Could you check a few things on this model? Use its own coordinates, in mm. A direction names the side the tool comes from. Coordinates: 2 decimals unless noted, no trailing zeros. Write each loop counter-clockwise with the first axis right and the second up, starting at its lowest first coordinate (ties: lowest second). Pieces come first, ordered by that corner, then holes.
Item 1: I want a section at A-A on z = -119. Please give me the cut outline in (x, y).
Item 2: If I drill on probe 1 along Z at (x, y) = (85.5, 527); probe 2 along Y at (x, z) = (212.5, -297.5), over which ranges is the centre line in solid material (lowest first)?
Item 3: I want a section at D-D on x = -209. Please give me the cut outline in (y, z), then the cut area to 3 significant figures.
Item 4: I want a section at C-C on x = 107. Please give me the cut outline in (y, z), then the cut area to 3 significant figures.
Item 5: I want a section at B-B on y = 388. Please give me the cut outline in (x, z).
Item 6: Thinking about a two-plate mould opening in Y: for faces 5 (the flat face through (190.5, 27, -150)), 6 (the flat face through (3, 313, 330.2)), 7 (the flat face through (3, 313, -330.2)), 8 (the flat face through (-218, 0, 5)), which applies, +Y half, -Y half, draft (parallel to the pull), parting line (faces both ways), or undercut?
Item 7: Which directions (+Z, -Z, +X, -X, +Y, -Y) give clear straight access to the entire face, cutting with the end or side of a thin tool? Please do faces 1 (the flat face through (-190.5, 611, 201)), 2 (the flat face through (216, 588.496, -155)), 3 (the flat face through (3, 313, 25.4)), 4 (the flat face through (3, 313, 381)).
from build123d import *

# Parameters (mm, degrees)
F0_W     = 381
F0_H     = 50.8
F0_W_2   = 50.8
F1_DEPTH = 635
F2_W     = 533.4
F2_H     = 254
F2_H_2   = 355.6
F3_DEPTH = 482.601


with BuildPart() as f1:
    # F0 (on Front) → F1 (new body)
    with BuildSketch(Plane.XZ):
        with Locations((0, 355.6)):
            Rectangle(F0_W, F0_H)
        Polygon((241.3, 381), (190.5, 381), (190.5, 330.2), (190.5, 76.2), (241.3, 76.2), align=None)
        Polygon((241.3, 25.4), (190.5, 25.4), (190.5, -330.2), (190.5, -381), (241.3, -381), align=None)
        with Locations((0, -355.6)):
            Rectangle(F0_W, F0_H)
        Polygon((-190.5, 381), (-241.3, 381), (-241.3, 76.2), (-190.5, 76.2), (-190.5, 330.2), align=None)
        Polygon((-190.5, 25.4), (-241.3, 25.4), (-241.3, -381), (-190.5, -381), (-190.5, -330.2), align=None)
        with Locations((0, 50.8)):
            Rectangle(F0_W, F0_H)
        with Locations((-215.9, 50.8)):
            Rectangle(F0_W_2, F0_H)
        with Locations((215.9, 50.8)):
            Rectangle(F0_W_2, F0_H)
    extrude(amount=-F1_DEPTH)

    # F2 (on face) → F3 (cut, through all)
    with BuildSketch(Plane.YZ.offset(241.3)):
        with Locations((321.7956796288, 203.2)):
            Rectangle(F2_W, F2_H)
        with Locations((321.7956796288, -152.4)):
            Rectangle(F2_W, F2_H_2)
    extrude(amount=-F3_DEPTH, mode=Mode.SUBTRACT)


solid = f1.part
Response values:
1. outline: (-241.3, 0) - (-190.5, 0) - (-190.5, 55.1) - (-241.3, 55.1) - close; (-241.3, 588.5) - (-190.5, 588.5) - (-190.5, 635) - (-241.3, 635) - close; (190.5, 0) - (241.3, 0) - (241.3, 55.1) - (190.5, 55.1) - close; (190.5, 588.5) - (241.3, 588.5) - (241.3, 635) - (190.5, 635) - close
2. probe 1: z = -381 to -330.2, 25.4 to 76.2, 330.2 to 381
2. probe 2: y = 0 to 55.1, 588.5 to 635
3. outline: (0, -381) - (635, -381) - (635, 381) - (0, 381) - close; hole (55.1, -330.2) - (588.5, -330.2) - (588.5, 25.4) - (55.1, 25.4) - close; hole (55.1, 76.2) - (588.5, 76.2) - (588.5, 330.2) - (55.1, 330.2) - close
3. area: 159,000 mm2
4. outline: (0, -381) - (635, -381) - (635, -330.2) - (0, -330.2) - close; (0, 25.4) - (635, 25.4) - (635, 76.2) - (0, 76.2) - close; (0, 330.2) - (635, 330.2) - (635, 381) - (0, 381) - close
4. area: 96,800 mm2
5. outline: (-241.3, -381) - (241.3, -381) - (241.3, -330.2) - (-241.3, -330.2) - close; (-241.3, 25.4) - (241.3, 25.4) - (241.3, 76.2) - (-241.3, 76.2) - close; (-241.3, 330.2) - (241.3, 330.2) - (241.3, 381) - (-241.3, 381) - close
6. face 5: draft
6. face 6: undercut
6. face 7: undercut
6. face 8: -Y half
7. face 1: +Y, -Y
7. face 2: +X, -X
7. face 3: none
7. face 4: +Z, +X, -X, +Y, -Y
